Design review of the part built by this model. Coordinates are the model's own, in mm. Face numbers are marked on the shaded views. A direction names the side the tool comes from. Round coordinates to 2 decimals unless told otherwise and drop trailing zeros. Loops run counter-clockwise (first coordinate to the right, second up) from the corner with the lowest first, then second, coordinate; pieces in that order, holes last. Notation, with made-up numbers: (40.5, 74) - (69.5, 74) arc R30 cw to (69.5, 108) - close; hole circle Ø6 at (-10.5, -39). An arc over 180 degrees is marked (long way). Use one line per item in the form item = value. Start each with the question number.
(1) Machinability: for the marked faces 4, 5, 6, 7 and 8, which of the approach directions +Z, -Z, +X, -X, +Y, -Y give a long, thin tool a straight path to every point of the face, cutting with its end or side? Answer none if there is none.
(2) We need section A-A, the plane x = 45. Write out the cut boundary in (y, z).
(3) We need section C-C, the plane x = 100.5. Write out the cut boundary in (y, z), then the cut area to 3 significant figures.
(4) Wall thickness on probe 1 along Y at (x, z) = (101.5, 0); probe 2 along Y at (x, z) = (89.5, -1.5); probe 3 along X at (y, z) = (-50.5, -13): over which ranges is each line inside the solid? List them lowest first. Write a range as [from, to].
(5) The part is to be moulded in two halves that separate along X. For the marked faces 1, 2 and 3, say which applies: released by +X, released by -X, zero draft, split by the parting line, or undercut.
(6) For pin 1 (3 mm diameter, centred on y = 49.5, z = 23.5, fed in from +X); pin 2 (23 mm diameter, centred on y = -9, z = -4.5, fed in from +X); pin 3 (5 mm diameter, centred on x = 21, y = -11, fed in from +Z); pin 4 (5 mm diameter, centred on y = -26, z = 32, fed in from -X), all flat-tipped, find the tip position at first contact; note any pin that passes through.
(7) We need section B-B, the plane x = 12. Write out the cut boundary in (y, z), then the cut area to 3 significant figures.
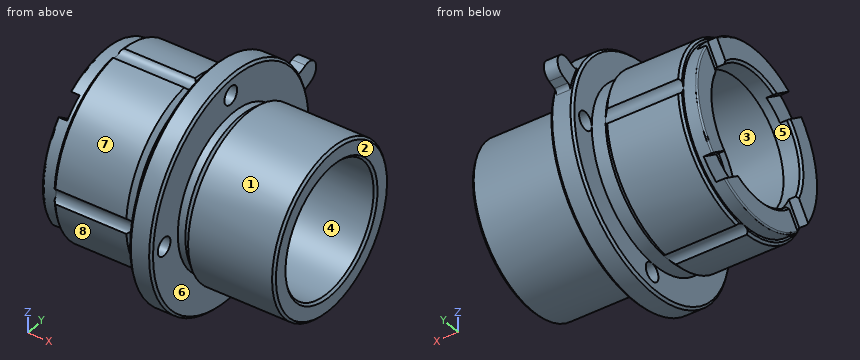
from build123d import *

# Parameters (mm, degrees)
CHAMFER1_SIZE       = 1.27
FILLET1_R           = 0.762
SKETCH2_R           = 5.08
CUT_EXTRUDE1_DEPTH  = 115.553718465
CIRPATTERN1_COUNT   = 4
CUT_EXTRUDE2_DEPTH  = 5.08
CIRPATTERN2_COUNT   = 4
BOSS_EXTRUDE1_DEPTH = 7.62
FILLET2_R           = 2.54


with BuildPart() as part:
    # Sketch1 → Base-Revolve (revolve)
    with BuildSketch(Plane.XY, mode=Mode.PRIVATE) as base_revolve_sk:
        Polygon((0, 35.56), (0, 48.26), (7.62, 48.26), (7.62, 50.8), (48.26, 50.8), (50.8, 48.26), (58.42, 48.26), (58.42, 63.5), (71.12, 63.5), (71.12, 42.416108007), (75.319090909, 42.416108007), (79.129090909, 45.72), (127, 45.72), (127, 35.56), (83.82, 35.56), (81.915, 33.02), (63.5, 33.02), (63.5, 30.48), (38.1, 30.48), (38.1, 38.1), (10.16, 38.1), (10.16, 35.56), align=None)
    revolve(base_revolve_sk.sketch.rotate(Axis((0, 0, 0), (1, 0, 0)), 90), axis=Axis((0, 0, 0), (1, 0, 0)))

    # Chamfer1
    chamfer1_edges = [part.edges().sort_by_distance(p)[0] for p in [
        (38.1, 0, -30.48),
        (127, 0, -35.56),
        (127, 0, -45.72),
        (71.12, 0, -63.5),
        (58.42, 0, -63.5),
        (7.62, 0, -50.8),
        (0, 0, -35.56),
    ]]
    chamfer(chamfer1_edges, length=CHAMFER1_SIZE)

    # Fillet1
    fillet1_edges = [part.edges().sort_by_distance(p)[0] for p in [
        (0, 0, -48.26),
    ]]
    fillet(fillet1_edges, radius=FILLET1_R)

    # Sketch2 → Cut-Extrude1 (cut, through all)
    with BuildSketch(Plane(origin=(71.12, 0, 0), x_dir=(0, 0, -1), z_dir=(1, 0, 0))):
        with Locations((53.34, 0)):
            Circle(SKETCH2_R)
    cut_extrude1 = extrude(amount=-CUT_EXTRUDE1_DEPTH, mode=Mode.SUBTRACT)

    # CirPattern1: Cut-Extrude1 ×4 about axis
    cirpattern1_axis = Axis((0, 0, 0), (1, 0, 0))
    for i in range(1, CIRPATTERN1_COUNT):
        add(cut_extrude1.rotate(cirpattern1_axis, i * 360 / CIRPATTERN1_COUNT), mode=Mode.SUBTRACT)

    # Sketch5 → Cut-Extrude2 (cut)
    with BuildSketch(Plane.ZY):
        Polygon((45.72, 55.88), (53.34, 45.72), (10.668, 13.716), (3.048, 23.876), align=None)
    cut_extrude2 = extrude(amount=-CUT_EXTRUDE2_DEPTH, mode=Mode.SUBTRACT)

    # CirPattern2: Cut-Extrude2 ×4 about axis
    cirpattern2_axis = Axis((0, 0, 0), (1, 0, 0))
    for i in range(1, CIRPATTERN2_COUNT):
        add(cut_extrude2.rotate(cirpattern2_axis, i * 360 / CIRPATTERN2_COUNT), mode=Mode.SUBTRACT)

    # Sketch7 → Boss-Extrude1 (add)
    with BuildSketch(Plane(origin=(68.58, 0, 0), x_dir=(0, 0, -1), z_dir=(1, 0, 0))):
        with BuildLine():
            Line((-29.857155153, 63.465701652), (-27.576463003, 57.199551469))
            ThreePointArc((-27.576463003, 57.199551469), (-21.718279101, 59.67048142), (-15.642366719, 61.543207289))
            Line((-15.642366719, 61.543207289), (-17.923058869, 67.809357472))
            ThreePointArc((-17.923058869, 67.809357472), (-26.061934921, 71.604577704), (-29.857155153, 63.465701652))
        make_face()
    extrude(amount=-BOSS_EXTRUDE1_DEPTH)

    # Fillet2
    fillet2_edges = [part.edges().sort_by_distance(p)[0] for p in [
        (64.77, 61.543207289, 15.642366719),
        (64.77, 57.199551469, 27.576463003),
    ]]
    fillet(fillet2_edges, radius=FILLET2_R)


solid = part.part
Data:
q1.face_4 = +X
q1.face_5 = -X
q1.face_6 = none
q1.face_7 = +Z, -X, -Y
q1.face_8 = -Z, -X, -Y
q2.outline = (-50.62, -4.29) arc R50.8 ccw to (-4.29, -50.62) arc R5.08 cw to (4.29, -50.62) arc R50.8 ccw to (50.62, -4.29) arc R5.08 cw to (50.62, 4.29) arc R50.8 ccw to (4.29, 50.62) arc R5.08 cw to (-4.29, 50.62) arc R50.8 ccw to (-50.62, 4.29) arc R5.08 cw to start; hole circle Ø60.96 at (0, 0)
q3.outline = circle Ø91.44 at (0, 0); hole circle Ø71.12 at (0, 0)
q3.area = 2,590 mm^2
q4.probe_1 = [-45.72, -35.56], [35.56, 45.72]
q4.probe_2 = [-45.7, -35.53], [35.53, 45.7]
q4.probe_3 = [58.42, 71.12]
q5.face_1 = zero draft
q5.face_2 = released by +X
q5.face_3 = undercut
q6.pin_1 = 71.12
q6.pin_2 = through
q6.pin_3 = 50.08
q6.pin_4 = 5.08
q7.outline = (-50.62, -4.29) arc R50.8 ccw to (-4.29, -50.62) arc R5.08 cw to (4.29, -50.62) arc R50.8 ccw to (50.62, -4.29) arc R5.08 cw to (50.62, 4.29) arc R50.8 ccw to (4.29, 50.62) arc R5.08 cw to (-4.29, 50.62) arc R50.8 ccw to (-50.62, 4.29) arc R5.08 cw to start; hole circle Ø76.2 at (0, 0)
q7.area = 3,490 mm^2
